Autodesk Inventor part; units mm, degrees
ref_plane "YZ Plane" through (0, 0, 0) normal (1, 0, 0) x (0, 1, 0)
ref_plane "XZ Plane" through (0, 0, 0) normal (0, 1, 0) x (-1, 0, 0)
ref_plane "XY Plane" through (0, 0, 0) normal (0, 0, 1) x (1, 0, 0)
sketch "Sketch1" plane through (0, 0, 0) normal (0, 1, 0) x (-1, 0, 0)
  line L0 (9.0944, 11.3049) -> (-22.9063, 11.3049)
  line L1 (9.0944, 11.3049) -> (41.0951, 11.3049) construction
  line L2 (-22.9063, 11.3049) -> (-22.9063, -19.1751)
  line L3 (-22.9063, -19.1751) -> (9.0944, -19.1751)
  line L4 (9.0944, -19.1751) -> (9.0944, 11.3049)
  point P0 (0, 0)
  dimension "d0" = 32.0007
  dimension "d1" = 180
  dimension "d2" = 30.48
extrude "Extrusion1" add sketch "Sketch1" along normal blind 2
sketch "Sketch2" plane through (0, 2, 0) normal (0, 1, 0) x (1, 0, 0)
  line L0 (-9.0944, 19.1751) -> (-9.0944, -11.3049)
  line L1 (-9.0944, -11.3049) -> (-9.0944, -10.3049)
  line L2 (-9.0944, -10.3049) -> (-8.0944, -10.3049)
  line L3 (-9.0944, 19.1751) -> (-8.0944, 19.1751)
  line L4 (22.9063, 19.1751) -> (-9.0944, 19.1751)
  line L5 (-8.0944, 19.1751) -> (-8.0944, 18.1751)
  line L6 (22.9063, 19.1751) -> (21.9063, 19.1751)
  line L7 (21.9063, 19.1751) -> (21.9063, 18.1751)
  line L8 (22.9063, -11.3049) -> (22.9063, 19.1751)
  line L9 (22.9063, -11.3049) -> (22.9063, -10.3049)
  line L10 (21.9063, -10.3049) -> (22.9063, -10.3049)
  line L11 (-8.0944, -10.3049) -> (21.9063, -10.3049)
  line L12 (21.9063, -10.3049) -> (21.9063, 18.1751)
  line L13 (21.9063, 18.1751) -> (-8.0944, 18.1751)
  line L14 (-8.0944, 18.1751) -> (-8.0944, -10.3049)
  line L15 (-9.0944, -11.3049) -> (22.9063, -11.3049)
  line L16 (22.9063, -11.3049) -> (22.9063, 19.1751)
  line L17 (22.9063, 19.1751) -> (-9.0944, 19.1751)
  line L18 (-9.0944, 19.1751) -> (-9.0944, -11.3049)
  line L19 (22.9063, -11.3049) -> (22.9063, -3.3649)
  line L20 (22.9063, 19.1751) -> (22.9063, 11.2351)
  line L21 (22.9063, -3.3649) -> (21.9063, -3.3649)
  line L22 (22.9063, 11.2351) -> (21.9063, 11.2351)
  point P0 (0, 0)
  point P1 (22.9063, -3.3649)
  point P2 (22.9063, 11.2351)
  dimension "d5" = 1
  dimension "d6" = 1
  dimension "d7" = 1
  dimension "d8" = 1
  dimension "d11" = 7.94
  dimension "d12" = 7.94
extrude "Extrusion3" add sketch "Sketch2" along normal blind 20 contours L3 L5 L14 L2 L0 | L2 L11 L10 L8 L15 L0 | L4 L7 L13 L5 | L4 L8 L22 L12 L7 | L12 L21 L8 L10
sketch "Sketch3" plane through (0, 2, 0) normal (0, 1, 0) x (1, 0, 0)
  line L0 (21.9063, -10.3049) -> (21.9063, -3.3649)
  line L1 (22.9063, 11.2351) -> (21.9063, 11.2351)
  line L2 (21.9063, -3.3649) -> (21.9063, 11.2351)
  line L3 (21.9063, 11.2351) -> (22.9063, 11.2351)
  line L4 (22.9063, -3.3649) -> (22.9063, 11.2351)
  line L5 (22.9063, 11.2351) -> (22.9063, -3.3649)
  line L6 (22.9063, -3.3649) -> (21.9063, -3.3649)
  point P0 (0, 0)
extrude "Extrusion4" add sketch "Sketch3" along normal blind 2
sketch "Sketch4" plane through (0, 22, 0) normal (0, 1, 0) x (1, 0, 0)
  line L0 (22.9063, -11.3049) -> (22.9063, 19.1751)
  line L1 (22.9063, 3.9351) -> (5.9063, 3.9351)
  line L2 (5.9063, 3.9351) -> (5.9063, 21.4351)
  line L3 (5.9063, 21.4351) -> (5.9063, -13.5649)
  circle A0 centre (5.9063, -13.5649) radius 2
  circle A1 centre (5.9063, 21.4351) radius 2
  line L4 (22.9063, 19.1751) -> (-9.0944, 19.1751)
  line L5 (5.9063, 19.1751) -> (2.4063, 19.1751)
  line L6 (2.4063, 19.1751) -> (2.4063, 24.1751)
  line L7 (2.4063, 24.1751) -> (9.4063, 24.1751)
  line L8 (9.4063, 24.1751) -> (9.4063, 19.1751)
  line L9 (9.4063, -11.3049) -> (9.4063, -16.3049)
  line L10 (9.4063, -16.3049) -> (2.4063, -16.3049)
  line L11 (2.4063, -16.3049) -> (2.4063, -11.3049)
  line L12 (-9.0944, -11.3049) -> (22.9063, -11.3049)
  point P0 (0, 0)
  dimension "d17" = 17
  dimension "d18" = 17.5
  dimension "d19" = 35
  dimension "d20" = 4
  dimension "d21" = 4
  dimension "d22" = 3.5
  dimension "d23" = 5
  dimension "d24" = 7
  dimension "d25" = 5
extrude "Extrusion5" add sketch "Sketch4" against normal blind 4 contours L9 L10 L11 L12 | L4 L6 L7 L8
sketch "Sketch5" plane through (0, 22, 0) normal (0, 1, 0) x (1, 0, 0)
  line L0 (2.4063, 19.1751) -> (2.4063, 24.1751)
  line L1 (2.4063, 19.1751) -> (2.4063, 18.1751)
  line L2 (-8.0944, 18.1751) -> (21.9063, 18.1751)
  line L3 (22.9063, 19.1751) -> (9.4063, 19.1751)
  line L4 (9.4063, 19.1751) -> (9.4063, 18.1751)
  line L5 (-9.0944, -11.3049) -> (22.9063, -11.3049)
  line L6 (2.4063, -11.3049) -> (2.4063, -10.3049)
  line L7 (-8.0944, -10.3049) -> (21.9063, -10.3049)
  line L8 (9.4063, -10.3049) -> (9.4063, -11.3049)
  circle A0 centre (5.9063, 21.4351) radius 2
  circle A1 centre (5.9063, -13.5649) radius 2
  line L9 (21.9063, -10.3049) -> (-8.0944, -10.3049)
  line L10 (-8.0944, -10.3049) -> (-8.0944, 18.1751)
  line L11 (-8.0944, 18.1751) -> (21.9063, 18.1751)
  line L12 (21.9063, 18.1751) -> (21.9063, 11.2351)
  line L13 (21.9063, 11.2351) -> (22.9063, 11.2351)
  line L14 (22.9063, 11.2351) -> (22.9063, 19.1751)
  line L15 (22.9063, 19.1751) -> (9.4063, 19.1751)
  line L16 (9.4063, 19.1751) -> (9.4063, 24.1751)
  line L17 (9.4063, 24.1751) -> (2.4063, 24.1751)
  line L18 (2.4063, 24.1751) -> (2.4063, 19.1751)
  line L19 (2.4063, 19.1751) -> (-9.0944, 19.1751)
  line L20 (-9.0944, 19.1751) -> (-9.0944, -11.3049)
  line L21 (-9.0944, -11.3049) -> (2.4063, -11.3049)
  line L22 (2.4063, -11.3049) -> (2.4063, -16.3049)
  line L23 (2.4063, -16.3049) -> (9.4063, -16.3049)
  line L24 (9.4063, -16.3049) -> (9.4063, -11.3049)
  line L25 (9.4063, -11.3049) -> (22.9063, -11.3049)
  line L26 (22.9063, -11.3049) -> (22.9063, -3.3649)
  line L27 (22.9063, -3.3649) -> (21.9063, -3.3649)
  line L28 (21.9063, -3.3649) -> (21.9063, -10.3049)
  point P0 (0, 0)
  point P1 (-8.0944, 18.1751)
  point P2 (22.9063, 19.1751)
extrude "Extrusion6" add sketch "Sketch5" along normal blind 2 contours L1 L2 L10 L7 L6 L5 L20 L19 | L4 L3 L14 L13 L12 L2 | L8 L7 L28 L27 L26 L5
sketch "Sketch35" plane through (-9.0944, 0, 11.3049) normal (0, 0, 1) x (1, 0, 0)
  line L0 (32.0007, 0) -> (32.0007, 24)
  line L1 (32.0007, 12) -> (32.0007, 32)
  line L2 (32.0007, 32) -> (67.0007, 32)
  line L3 (67.0007, 32) -> (67.0007, -8)
  line L4 (67.0007, -8) -> (32.0007, -8)
  line L5 (32.0007, -8) -> (32.0007, 0)
  point P0 (9.0944, 0)
  dimension "d177" = 20
  dimension "d178" = 35
  dimension "d179" = 40
extrude "Extrusion32" add sketch "Sketch35" against normal blind 1
sketch "Sketch36" plane through (-9.0944, 0, 10.3049) normal (0, 0, -1) x (-1, 0, 0)
  line L0 (-32.0007, 32) -> (-32.0007, 24)
  line L1 (-32.0007, 32) -> (-37.0007, 32)
  line L2 (-32.0007, 32) -> (-67.0007, 32)
  line L3 (-37.0007, 32) -> (-37.0007, 27)
  line L4 (-37.0007, 27) -> (-37.0007, -2.6)
  line L5 (-37.0007, -2.6) -> (-63.0507, -2.6)
  line L6 (-63.0507, -2.6) -> (-63.0507, 27)
  point P0 (-9.0944, 0)
  dimension "d182" = 5
  dimension "d183" = 5
  dimension "d184" = 29.6
  dimension "d185" = 26.05
  dimension "d186" = 29.6
  dimension "d187" = 90
hole "Hole3" at (27.9063, 27, 10.3049) at (53.9563, 27, 10.3049) at (53.9563, -2.6, 10.3049) at (27.9063, -2.6, 10.3049) direction (0, 0, 1) diameter 3.4 end through all
sketch "Sketch37" plane through (-9.0944, 0, 10.3049) normal (0, 0, -1) x (-1, 0, 0)
  point P0 (-9.0944, 0)
sketch "Sketch38" plane through (2.4063, 18, 11.3049) normal (0, 0, 1) x (1, 0, 0)
  line L0 (20.5, -18) -> (20.5, 6)
  line L1 (19.5, -16) -> (19.5, 6)
  line L2 (20.5, 6) -> (19.5, 6)
  line L3 (19.5, 6) -> (19.5, 15)
  line L4 (19.5, 15) -> (56.5, 15)
  line L5 (56.5, 15) -> (56.5, -27)
  line L6 (56.5, -27) -> (19.5, -27)
  line L7 (19.5, -27) -> (19.5, 15)
  circle A0 centre (51.55, -20.6) radius 1.7
  circle A1 centre (25.5, 9) radius 1.7
  circle A2 centre (51.55, 9) radius 1.7
  circle A3 centre (25.5, -20.6) radius 1.7
  line L8 (0, 0) -> (0, 4)
  line L9 (0, 4) -> (0, 6)
  line L10 (-11.5007, 6) -> (0, 6)
  line L11 (-11.5007, -18) -> (-11.5007, 6)
  line L12 (-11.5007, -18) -> (20.5, -18)
  line L13 (20.5, -18) -> (20.5, -26)
  line L14 (20.5, -26) -> (55.5, -26)
  line L15 (55.5, -26) -> (55.5, 14)
  line L16 (55.5, 14) -> (20.5, 14)
  line L17 (20.5, 14) -> (20.5, 6)
  line L18 (7, 6) -> (20.5, 6)
  line L19 (7, 4) -> (7, 6)
  line L20 (7, 4) -> (7, 0)
  line L21 (7, 0) -> (0, 0)
  line L22 (20.5, 15) -> (21.5, 15)
  line L23 (21.5, 15) -> (21.5, 6)
  line L24 (20.5, 6) -> (20.5, 14)
  line L25 (21.5, 6) -> (20.5, 6)
  line L26 (20.5, -26) -> (21.5, -26)
  line L27 (55.5, -26) -> (20.5, -26)
  line L28 (21.5, -26) -> (21.5, -18)
  line L29 (20.5, -18) -> (-11.5007, -18)
  line L30 (21.5, -18) -> (20.5, -18)
  line L31 (20.5, -26) -> (20.5, -27)
  line L32 (20.5, 14) -> (20.5, 15)
  line L33 (19.5, -16) -> (19.5, 6)
  line L34 (19.5, 6) -> (19.5, 7)
  line L35 (19.5, 7) -> (20.5, 7)
  point P0 (-2.4063, -18)
  point P1 (19.5, 7)
  point P2 (20.5, 7)
  point P3 (19.5, -18)
  dimension "d195" = 1
  dimension "d196" = 9
  dimension "d197" = 37
  dimension "d198" = 42
  dimension "d199" = 1
  dimension "d200" = 1
  dimension "d201" = 1
extrude "Extrusion33" add sketch "Sketch38" against normal blind 30 contours L13 L31 L6 L7 L12 | L14 L15 L16 L23 L4 L5 L6 L31 | L35 L3 L4 L32 L17 | L32 L4 L23 L16
sketch "Sketch42" plane through (2.4063, 18, 11.3049) normal (0, 0, 1) x (1, 0, 0)
  circle A0 centre (25.5, 9) radius 1.7
  circle A1 centre (25.5, 9) radius 3.5
  circle A2 centre (51.55, 9) radius 1.7
  circle A3 centre (51.55, 9) radius 3.5
  circle A4 centre (51.55, -20.6) radius 1.7
  circle A5 centre (51.55, -20.6) radius 3.5
  circle A6 centre (25.5, -20.6) radius 1.7
  circle A7 centre (25.5, -20.6) radius 3.5
  circle A8 centre (51.55, -20.6) radius 1.7
  circle A9 centre (25.5, 9) radius 1.7
  circle A10 centre (51.55, 9) radius 1.7
  circle A11 centre (25.5, -20.6) radius 1.7
  line L0 (0, 0) -> (0, 4)
  line L1 (0, 4) -> (0, 6)
  line L2 (-11.5007, 6) -> (0, 6)
  line L3 (-11.5007, -18) -> (-11.5007, 6)
  line L4 (-11.5007, -18) -> (19.5, -18)
  line L5 (19.5, -18) -> (19.5, -27)
  line L6 (19.5, -27) -> (56.5, -27)
  line L7 (56.5, -27) -> (56.5, 15)
  line L8 (56.5, 15) -> (19.5, 15)
  line L9 (19.5, 15) -> (19.5, 7)
  line L10 (19.5, 7) -> (20.5, 7)
  line L11 (20.5, 7) -> (20.5, 6)
  line L12 (7, 6) -> (20.5, 6)
  line L13 (7, 4) -> (7, 6)
  line L14 (7, 4) -> (7, 0)
  line L15 (7, 0) -> (0, 0)
  line L16 (19.5, -14) -> (19.5, 6)
  line L17 (19.5, 6) -> (19.5, -18)
  line L18 (20.5, -18) -> (20.5, 6)
  line L19 (19.5, 15) -> (19.5, 7)
  line L20 (19.5, 7) -> (19.5, 6)
  point P0 (-2.4063, -18)
  dimension "d224" = 7
  dimension "d225" = 7
  dimension "d226" = 7
  dimension "d227" = 7
extrude "Extrusion37" add sketch "Sketch42" along normal blind 6 contours L20 L10 L11 L12 | L12 L11 L10 L9 L8 L7 L6 L5 L17 L16
extrude "Extrusion38" add sketch "Sketch38" against normal blind 8 contours L2 L3 L35 L17
properties part number "shell 3.0"
Can you work these out from the model? Positions are in its coordinate system, mm. A direction names the side the tool comes from. Coordinates: 2 decimals unless noted, no trailing zeros. Order: outer loops, then holes, each group sorted by start corner. A loop starts at its lowest first (then second) coordinate and runs counter-clockwise, first axis right, second up. Notation, with made-up numbers: M -20.5,69.5 L -16.5,69.5 A31 ccw -16.5,101.5 Z; hole C 48.5,-36 d3. An arc over 180 degrees is marked long. Write item = value, one per line.
(1) If we mould it in two halves opening along Y, with no side actions, what happens to faces 1 (the face through (57.906, 12, -4)), 2 (the face through (6.83, 20.03, -19.66)), 3 (the face through (4, 18, 15))? For each: pulls with the +Y half, pulls with the -Y half, needs draft (parallel to the pull), parting line crosses it, or undercut.
Results are:
face_1 = undercut
face_2 = needs draft
face_3 = pulls with the -Y half
(2) Suppose I cut it at A-A on y = -2.6. Please give me the cut outline in (x, z), plus the area to 3 significant figures.
Results are:
outline = M 21.91,-18.7 L 22.91,-18.7 L 22.91,10.3 L 26.21,10.3 L 26.21,11.3 L 24.41,11.3 L 24.41,17.3 L 21.91,17.3 Z; M 29.61,10.3 L 52.26,10.3 L 52.26,11.3 L 50.46,11.3 L 50.46,17.3 L 31.41,17.3 L 31.41,11.3 L 29.61,11.3 Z; M 55.66,10.3 L 57.91,10.3 L 57.91,-18.7 L 58.91,-18.7 L 58.91,17.3 L 57.46,17.3 L 57.46,11.3 L 55.66,11.3 Z
area = 226 mm2
(3) Suppose I cut it at D-D on y = 15. Please give me the cut outline in (x, z), plus the area to 3 significant figures.
Results are:
outline = M -9.09,-19.18 L 22.91,-19.18 L 22.91,-11.24 L 21.91,-11.24 L 21.91,-18.18 L -8.09,-18.18 L -8.09,10.3 L 21.91,10.3 L 21.91,3.36 L 22.91,3.36 L 22.91,10.3 L 57.91,10.3 L 57.91,-18.7 L 58.91,-18.7 L 58.91,17.3 L 21.91,17.3 L 21.91,11.3 L -9.09,11.3 Z
area = 393 mm2
(4) For faces 4 (the face through (9.406, 20, 14)), 5 (the face through (41, 32, -4)), 6 (the face through (7, 13, -18.175)), 7 (the face through (52, -3, 11.305)), which set-ups out of +Z, -Z, +X, -X, +Y, -Y let a thin tool reach every point of the face, with its end or its side?
Results are:
face_4 = +Z, +Y, -Y
face_5 = -Z
face_6 = +Y
face_7 = +Z
(5) I need wall thicknesses on line 1 along X through (y, z) = (27, 10.85); line 2 along X through (y, z) = (16.5, -5.5); line 3 along Y through (x, z) = (29.5, -18). Which ranges of each line are inside material? Lowest first, please. Write a range as [from, to].
Results are:
line_1 = [21.91, 26.21], [29.61, 52.26], [55.66, 58.91]
line_2 = [-9.09, -8.09], [57.91, 58.91]
line_3 = [-9, -8], [32, 33]
(6) Suppose I cut it at B-B on z = 6. Please give me the cut outline in (x, y).
Results are:
outline = M -9.09,0 L 21.91,0 L 21.91,-9 L 58.91,-9 L 58.91,33 L 21.91,33 L 21.91,2 L -8.09,2 L -8.09,24 L -9.09,24 Z; hole M 22.91,-8 L 57.91,-8 L 57.91,32 L 22.91,32 Z
(7) For pin 1 Ø4.5 at (x, y) = (53.96, -2.6) entering from -Z; pin 2 Ø9 at (x, y) = (53.96, 27) entering from -Z; pin 3 Ø8 at (x, z) = (16, -13.5) entering from +Y, each with a flat end and sliding along its axis, tell me the tip position at first contact or that it passes through.
Results are:
pin_1 = 10.3
pin_2 = -18.7
pin_3 = 2
(8) Suppose I cut it at C-C on x = 35. Please give me the cut outline in (y, z), plus the area to 3 significant figures.
Results are:
outline = M -9,-18.7 L -8,-18.7 L -8,10.3 L 32,10.3 L 32,-18.7 L 33,-18.7 L 33,17.3 L -9,17.3 Z
area = 352 mm2
